Input: part model. Units: mm. Frame: model coordinates. A direction names the side the tool comes from. Coordinates: 2 decimals unless noted, no trailing zeros. Write each loop counter-clockwise with the first axis right and the second up, starting at its lowest first coordinate (ties: lowest second). Pieces come first, ordered by that corner, then holes. Notation, with made-up numbers: (-37.5, 61.25) -> (0.5, 61.25) arc R29 ccw to (0.5, 81.25) -> close; hole circle Ø8 at (-31, -9.75). An arc over 180 degrees is marked (long way). One line per question, with ' | ' between items. Start each with the question number.
```python
from build123d import *

# Parameters (mm, degrees)
SKETCH1_R           = 4
SKETCH1_R_2         = 2.6
BOSS_EXTRUDE3_DEPTH = 11
SKETCH3_R           = 4
BOSS_EXTRUDE4_DEPTH = 2
SKETCH4_R           = 0.5
CUT_EXTRUDE1_DEPTH  = 1


with BuildPart() as part:
    # Sketch1 → Boss-Extrude3 (new body)
    with BuildSketch(Plane.XY):
        Circle(SKETCH1_R)
        Circle(SKETCH1_R_2, mode=Mode.SUBTRACT)
    extrude(amount=BOSS_EXTRUDE3_DEPTH)

    # Sketch3 → Boss-Extrude4 (add)
    with BuildSketch(Plane.XY.offset(11)):
        Circle(SKETCH3_R)
    extrude(amount=BOSS_EXTRUDE4_DEPTH)

    # Sketch4 → Cut-Extrude1 (cut)
    with BuildSketch(Plane.XY.offset(13)):
        Circle(SKETCH4_R)
    extrude(amount=-CUT_EXTRUDE1_DEPTH, mode=Mode.SUBTRACT)


solid = part.part
```
1) Section A-A, the plane y = 0. Return loops of the section in (x, z).
2) Section B-B, the plane x = 1.75. Return loops of the section in (y, z), then the cut area to 3 significant figures.
3) Access query for faces 1 (the face through (0, 0, 12)), 2 (the face through (1, 0, 13)), 3 (the face through (-0.338, 2.578, 5.423)). Directions: +Z, -Z, +X, -X, +Y, -Y. A direction counts if a zero-diameter tool reaches every point of the face in a straight line with its end or side. Return the directions, or none.
4) Section C-C, the plane z = 8. Return loops of the section in (x, y), then the cut area to 3 significant figures.
5) Ray query, line 1 (Y direction, x = 0, z = 12.4); line 2 (Y direction, x = 0, z = 6); line 3 (Z direction, x = 2, y = -0.75). Return the intervals inside material, ascending.
6) Pull-direction query (Y, two-part tool) for faces 4 (the face through (-0.867, -3.905, 6.409)), 5 (the face through (-0.108, -0.488, 12.507)), 6 (the face through (3, 0, 0)); classes: released by +Y, released by -Y, zero draft, split by the parting line, or undercut.
7) First-contact query: P1, Ø1.6, axis at x = 1, y = 1, coming from the -Z side; P2, Ø0.5, axis at x = 0, y = 0, coming from the +Z side; P3, Ø1, axis at y = 3, z = 2.5, coming from the -X side. Flat tips, straight axial feed; report the tip coordinate or a pass-through.
Answer block:
1) outline: (-4, 0) -> (-2.6, 0) -> (-2.6, 11) -> (2.6, 11) -> (2.6, 0) -> (4, 0) -> (4, 13) -> (0.5, 13) -> (0.5, 12) -> (-0.5, 12) -> (-0.5, 13) -> (-4, 13) -> close
2) outline: (-3.6, 0) -> (-1.92, 0) -> (-1.92, 11) -> (1.92, 11) -> (1.92, 0) -> (3.6, 0) -> (3.6, 13) -> (-3.6, 13) -> close | area: 51.2 mm2
3) face 1: +Z | face 2: +Z, +X, -X, +Y, -Y | face 3: -Z
4) outline: circle Ø8 at (0, 0); hole circle Ø5.2 at (0, 0) | area: 29.0 mm2
5) line 1: y = -4 to -0.5, 0.5 to 4 | line 2: y = -4 to -2.6, 2.6 to 4 | line 3: z = 11 to 13
6) face 4: split by the parting line | face 5: undercut | face 6: zero draft
7) P1: stops at z = 11 | P2: stops at z = 12 | P3: stops at x = -3.12
